Job drawing, mm, ordinate dimensions from the low corner. One solid piece. Round coordinates to 2 decimals unless told otherwise and drop trailing zeros. Loops run counter-clockwise (first coordinate to the right, second up) from the corner with the lowest first, then second, coordinate; pieces in that order, holes last. Notation, with made-up numbers: M 55,68.25 L 106,68.25 A4 cw 106,72.25 Z; hole C 78.5,27.5 d3. An arc over 180 degrees is marked long. Use a Markdown table: item, result. Add a question column.
(1) Flat gauge pins, fed straight in: P1, Ø1, axis at x = 29, y = 1.5, coming from the +Z side; P2, Ø1.5, axis at x = 32.5, y = 4.5, coming from the +Z side; P3, Ø3, axis at x = 43.5, y = 2, coming from the +Z side. Where does each tip first touch, or does it go through?
(2) Band-saw the part on C-C, the plane y = 2.6. Write the cut outline in (x, z).
(3) Band-saw the part on B-B, the plane x = 57. Write the cut outline in (y, z), and give its area (3 significant figures).
(4) Band-saw the part on D-D, the plane x = 76. Write the cut outline in (y, z), and give its area (3 significant figures).
(5) Band-saw the part on A-A, the plane z = 25. Write the cut outline in (x, y), and give its area (3 significant figures).
(6) Wall check: L1, parallel to X at y = 3.7, z = 16.5 (1 decimal); L2, parallel to Z at x = 41, y = 4.05; L3, parallel to X at y = 3, z = 44.5 (1 decimal). Give the ranges that are in metal, low to high.
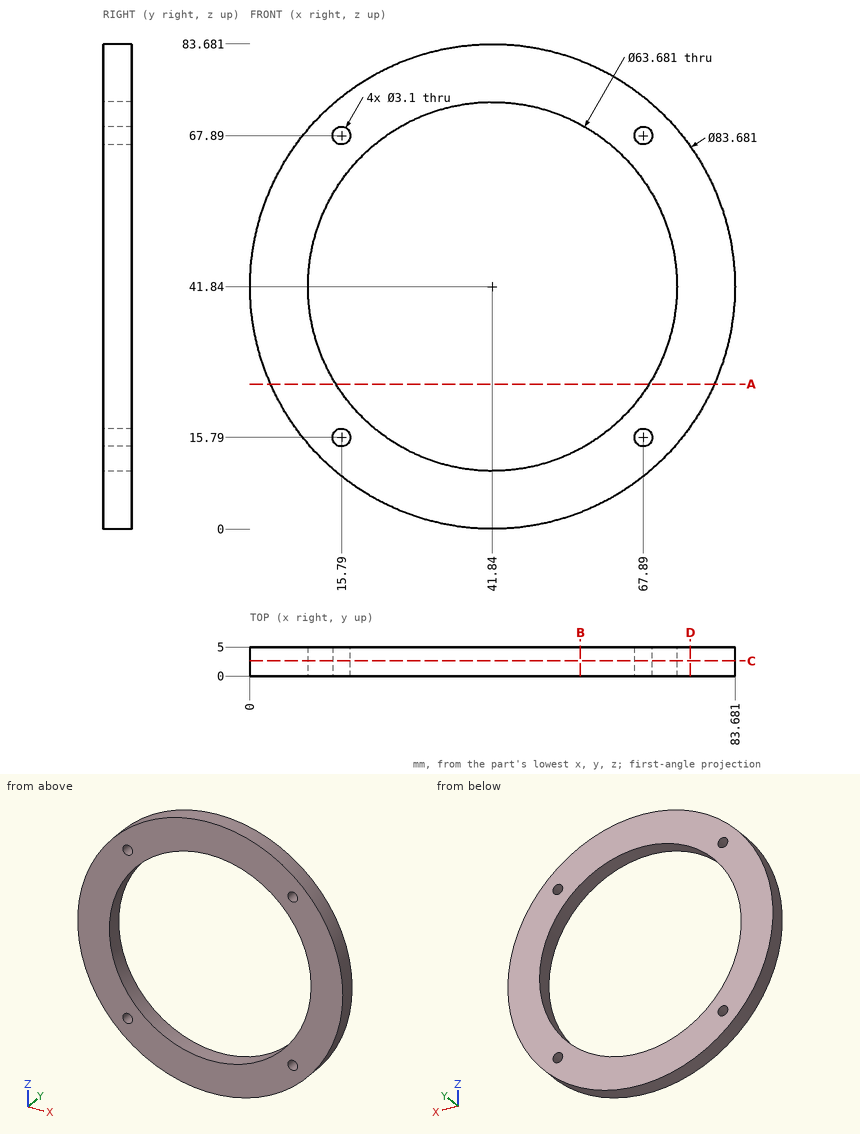
Return value:
| question | item | result |
|---|---|---|
| 1 | P1 | z = 81.82 |
| 1 | P2 | z = 82.79 |
| 1 | P3 | z = 83.68 |
| 2 | outline | C 41.84,41.84 d83.68; hole C 41.84,41.84 d63.68; hole C 15.79,15.79 d3.1; hole C 15.79,67.89 d3.1; hole C 67.89,15.79 d3.1; hole C 67.89,67.89 d3.1 |
| 3 | outline | M 0,2.84 L 5,2.84 L 5,13.84 L 0,13.84 Z; M 0,69.84 L 5,69.84 L 5,80.84 L 0,80.84 Z |
| 3 | area | 110 mm^2 |
| 4 | outline | M 0,17.68 L 5,17.68 L 5,66 L 0,66 Z |
| 4 | area | 242 mm^2 |
| 5 | outline | M 3.54,0 L 14.82,0 L 14.82,5 L 3.54,5 Z; M 68.86,0 L 80.14,0 L 80.14,5 L 68.86,5 Z |
| 5 | area | 113 mm^2 |
| 6 | L1 | 8.5 to 14.4, 17.2 to 22.6, 61.1 to 66.5, 69.3 to 75.1 |
| 6 | L2 | 0.01 to 10.01, 73.67 to 83.67 |
| 6 | L3 | 0.1 to 10.1, 73.6 to 83.6 |
